Input: part model. Units: mm. Frame: model coordinates. Face numbers are marked on the shaded views. Give positions to 0.01 mm unless a question says otherwise; leave off trailing zeros. Loops run counter-clockwise (first coordinate to the right, second up) from the corner with the lowest first, then second, coordinate; pieces in that order, holes last. Notation, with made-up numbers: M -31,2 L -2,2 A22 ccw -2,28 Z; hole C 41,-4 d10. An arc over 180 degrees is marked long. Use CSV: the item, a comma, the result in double quotes. Start each with the question number.
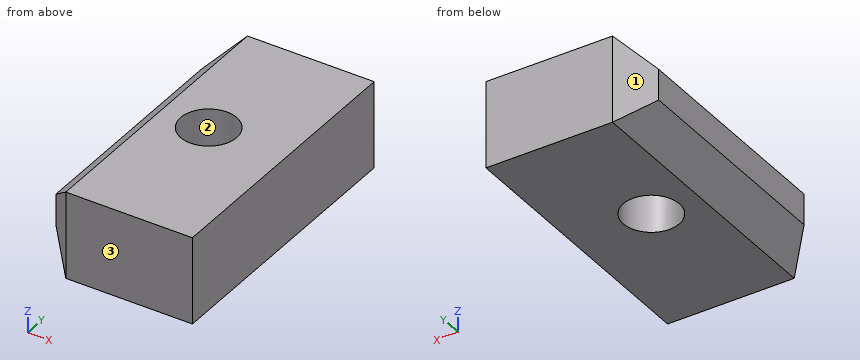
from build123d import *

# Parameters (mm, degrees)
F0_W     = 70.042707
F0_H     = 39.452329
F1_DEPTH = 127
F3_D     = 25.4
F4_SIZE  = 12.7


with BuildPart() as f1:
    # F0 (on Front) → F1 (new body)
    with BuildSketch(Plane.XZ):
        with Locations((35.021353, -19.726164)):
            Rectangle(F0_W, F0_H)
    extrude(amount=F1_DEPTH)

    # F3 (through all)
    with Locations(Plane.XY):
        with Locations((34.320448, -60.479335)):
            Hole(F3_D / 2)

    # F4
    f4_edges = [f1.edges().sort_by_distance(p)[0] for p in [
        (0, -63.5, 0),
        (0, -63.5, -39.452329),
        (0, 0, -19.726165),
        (0, -127, -19.726165),
    ]]
    chamfer(f4_edges, length=F4_SIZE)


solid = f1.part
Item 1: First-contact query: pin 1 Ø20.5 at (x, y) = (34.32, -60.48) entering from -Z; pin 2 Ø6 at (x, z) = (22, -7.5) entering from +Y. Flat tips, straight axial feed; report the tip coordinate or a pass-through.
Item 2: Section A-A (x = 28.5). Output: boundary loops of the cut face in (y, z).
Item 3: Mould query, pull axis Y, two halves, no side actions, for the marked faces 1, 2 and 3. Classes: +Y half, -Y half, draft (parallel to the pull), parting line (faces both ways), or undercut.
Item 4: Section C-C (z = -7.5). Output: boundary loops of the cut face in (x, y).
Item 5: Section D-D (y = -109). Output: boundary loops of the cut face in (x, z), then the cut area to 3 significant figures.
Item 6: Material intervals for line 1 (X direction, y = -65, z = -19.5); line 2 (Y direction, x = 45, z = -4); line 3 (Y direction, x = 43, z = -7), sorted ascending.
Item 7: Section B-B (y = -71). Output: boundary loops of the cut face in (x, z), then the cut area to 3 significant figures.
Recorded:
1,pin 1,"through"
1,pin 2,"y = 0"
2,outline,"M -127,-39.45 L -71.77,-39.45 L -71.77,0 L -127,0 Z; M -49.19,-39.45 L 0,-39.45 L 0,0 L -49.19,0 Z"
3,face 1,"+Y half"
3,face 2,"undercut"
3,face 3,"-Y half"
4,outline,"M 5.2,-119.5 L 12.7,-127 L 70.04,-127 L 70.04,0 L 12.7,0 L 5.2,-7.5 Z; hole C 34.32,-60.48 d25.4"
5,outline,"M 0,-26.75 L 12.7,-39.45 L 70.04,-39.45 L 70.04,0 L 12.7,0 L 0,-12.7 Z"
5,area,"2,600 mm²"
6,line 1,"0 to 22.45, 46.19 to 70.04"
6,line 2,"-127 to -67.35, -53.61 to 0"
6,line 3,"-127 to -69.75, -51.21 to 0"
7,outline,"M 0,-26.75 L 12.7,-39.45 L 27.21,-39.45 L 27.21,0 L 12.7,0 L 0,-12.7 Z; M 41.43,-39.45 L 70.04,-39.45 L 70.04,0 L 41.43,0 Z"
7,area,"2,040 mm²"
